For this review, use the dimensioned drawing (mm, ordinates from the lowest corner) and the shaded views. A direction names the side the tool comes from. Round coordinates to 2 decimals unless told otherwise and drop trailing zeros. Order: outer loops, then holes, each group sorted by start corner. A loop starts at its lowest first (then second) coordinate and runs counter-clockwise, first axis right, second up. Notation, with made-up numbers: (-26.75, 89) - (-4.75, 89) arc R23 ccw to (-4.75, 98) - close; hole circle Ø11 at (-29.5, 24.5). An arc over 180 degrees is marked (long way). Write item = value, one per line.
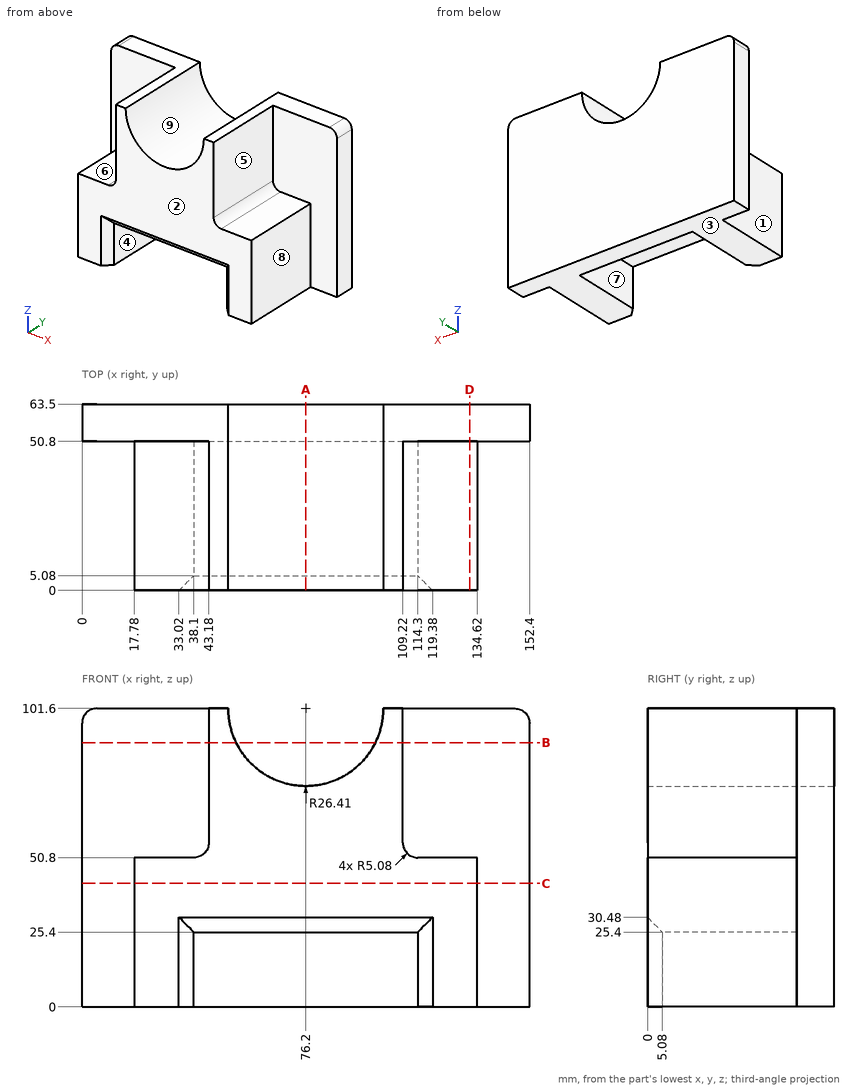
Item 1: For line 1 along X through (y, z) = (8, 9.5); line 2 along X through (y, z) = (33.5, 38); line 3 along Z through (x, y) = (22, 41), list the stretches that pass through material, from the lowest coordinate up. Write a range as [from, to].
Data:
line_1 = [17.78, 38.1], [114.3, 134.62]
line_2 = [17.78, 134.62]
line_3 = [0, 50.8]
Item 2: Take a section at D-D, the plane x = 132. State the section outline as (y, z) points, and give its area (3 significant figures).
Data:
outline = (0, 0) - (63.5, 0) - (63.5, 101.6) - (50.8, 101.6) - (50.8, 50.8) - (0, 50.8) - close
area = 3,870 mm2
Item 3: Take a section at A-A, the plane x = 76.2. State the section outline as (y, z) points.
Data:
outline = (0, 30.48) - (5.08, 25.4) - (50.8, 25.4) - (50.8, 0) - (63.5, 0) - (63.5, 75.19) - (0, 75.19) - close
Item 4: Take a section at C-C, the plane z = 42. State the section outline as (x, y) points, and give its area (3 significant figures).
Data:
outline = (0, 50.8) - (17.78, 50.8) - (17.78, 0) - (134.62, 0) - (134.62, 50.8) - (152.4, 50.8) - (152.4, 63.5) - (0, 63.5) - close
area = 7,870 mm2
Item 5: Take a section at B-B, the plane z = 90. State the section outline as (x, y) points.
Data:
outline = (0, 50.8) - (43.18, 50.8) - (43.18, 0) - (52.47, 0) - (52.47, 63.5) - (0, 63.5) - close; (99.93, 0) - (109.22, 0) - (109.22, 50.8) - (152.4, 50.8) - (152.4, 63.5) - (99.93, 63.5) - close
Item 6: Insertion check: P1, Ø3, axis at x = 101, z = 30, coming from the -Y side; P2, Ø8, axis at x = 83.5, y = 26, coming from the -Z side; P3, Ø13, axis at x = 132.5, z = 63, coming from the -Y side; P4, Ø6, axis at x = 23.5, y = 31.5, coming from the +Z side. Each pin has a flat end and moves straight along its axis. Give the tip position at first contact, or say it passes through.
Data:
P1 = 0
P2 = 25.4
P3 = 50.8
P4 = 50.8
Item 7: The part is to be moulded in two halves that separate along X. For the marked faces 6, 7, 8 and 9, say which applies: +X half, -X half, draft (parallel to the pull), parting line (faces both ways), or undercut.
Data:
face_6 = draft
face_7 = undercut
face_8 = +X half
face_9 = undercut
Item 8: For the marked faces 1, 2, 3, 4 and 5, list the 3-axis set-ups (+Z, -Z, +X, -X, +Y, -Y) from which the entire face can be reached by the end or side of a thin tool; tool diameter is ignored.
Data:
face_1 = +Z, -Z, -X, -Y
face_2 = +Z, -Z, +X, -X, -Y
face_3 = -Z, +X, -X, +Y, -Y
face_4 = -Z, -Y
face_5 = +Z, +X, -Y
